from build123d import *

# Parameters (mm, degrees)
F1_R     = 2.75
F1_R_2   = 1.5
F2_DEPTH = 2
F3_START = 1.5
F3_DEPTH = 0.5
F4_START = 2
F4_DEPTH = 21
F5_SIZE2 = 1.25
F5_SIZE  = 1.25
F6_R     = 0.25


# Not quite as in the source:
# - a feature names something its author has since deleted; it is built from what else it names


with BuildPart() as f2:
    # F1 (on Top) → F2 (new body)
    with BuildSketch(Plane.XY):
        Circle(F1_R)
        Circle(F1_R_2, mode=Mode.SUBTRACT)
        Circle(F1_R_2)
        Polygon((-0.5773502692, -1), (-1.1547005384, 0), (-0.5773502692, 1), (0.5773502692, 1), (1.1547005384, 0), (0.5773502692, -1), align=None, mode=Mode.SUBTRACT)
    extrude(amount=F2_DEPTH)

    # F1 (on Top) → F3 (join)
    with BuildSketch(Plane.XY.offset(F3_START)):
        Polygon((-0.5773502692, 1), (-1.1547005384, 0), (-0.5773502692, -1), (0.5773502692, -1), (1.1547005384, 0), (0.5773502692, 1), align=None)
    extrude(amount=F3_DEPTH)

    # F1 (on Top) → F4 (join)
    with BuildSketch(Plane.XY.offset(F4_START)):
        Circle(F1_R_2)
        Polygon((-0.5773502692, -1), (-1.1547005384, 0), (-0.5773502692, 1), (0.5773502692, 1), (1.1547005384, 0), (0.5773502692, -1), align=None, mode=Mode.SUBTRACT)
        Polygon((-0.5773502692, 1), (-1.1547005384, 0), (-0.5773502692, -1), (0.5773502692, -1), (1.1547005384, 0), (0.5773502692, 1), align=None)
    extrude(amount=F4_DEPTH)

    # F5
    f5_edges = [f2.edges().sort_by_distance(p)[0] for p in [
        (-2.75, 0, 0),
    ]]
    chamfer(f5_edges, length=F5_SIZE, length2=F5_SIZE2)

    # F6
    f6_edges = [f2.edges().sort_by_distance(p)[0] for p in [
        (-2.75, 0, 2),
        (-1.5, 0, 2),
        (-1.5, 0, 0),
        (-2.75, 0, 1.25),
    ]]
    fillet(f6_edges, radius=F6_R)


solid = f2.part
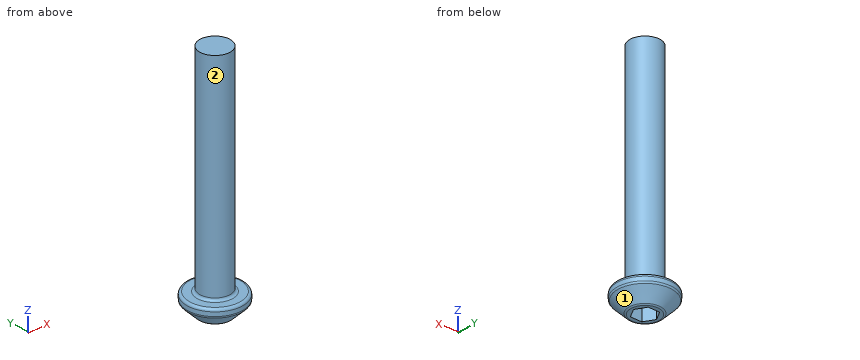
Read the model definition and answer for the solid it produces. Units are mm, in the model's axes. Face numbers are marked on the shaded views. A direction names the side the tool comes from. Round coordinates to 2 decimals unless told otherwise and drop trailing zeros. Write each loop counter-clockwise with the first axis right and the second up, starting at its lowest first coordinate (ties: lowest second). Pieces come first, ordered by that corner, then holes.
1. Straight lines are drawn through the part: L1, parallel to Y at x = -0.15, z = 1; L2, parallel to Y at x = 0.05, z = 4.5; L3, parallel to Z at x = 1.75, y = -1.55. For each, find the intervals that lie inside material, in ascending order.
2. Which of the six approach directions +Z, -Z, +X, -X, +Y, -Y give full straight-line access (tool end or side, diameter ignored) to the marked faces 1 and 2?
3. The part is cut by section A-A, the plane z = 10. Determine the outline of the cut face in (x, y).
4. Given pin 1 Ø2 at (x, z) = (1.5, 14) entering from +Y; pin 2 Ø2 at (y, z) = (2, 10.5) entering from +X; pin 3 Ø0.6 at (x, z) = (0, 0.5) entering from +Y, each flat-ended and moving along its own axis, determine where each tip first touches the part or whether it passes through.
Values:
1. L1: y = -2.5 to -1, 1 to 2.5
1. L2: y = -1.5 to 1.5
1. L3: z = 0.84 to 2
2. face 1: -Z
2. face 2: +Z
3. outline: circle Ø3 at (0, 0)
4. pin 1: stops at y = 1.41
4. pin 2: stops at x = 1.12
4. pin 3: stops at y = 2.3
